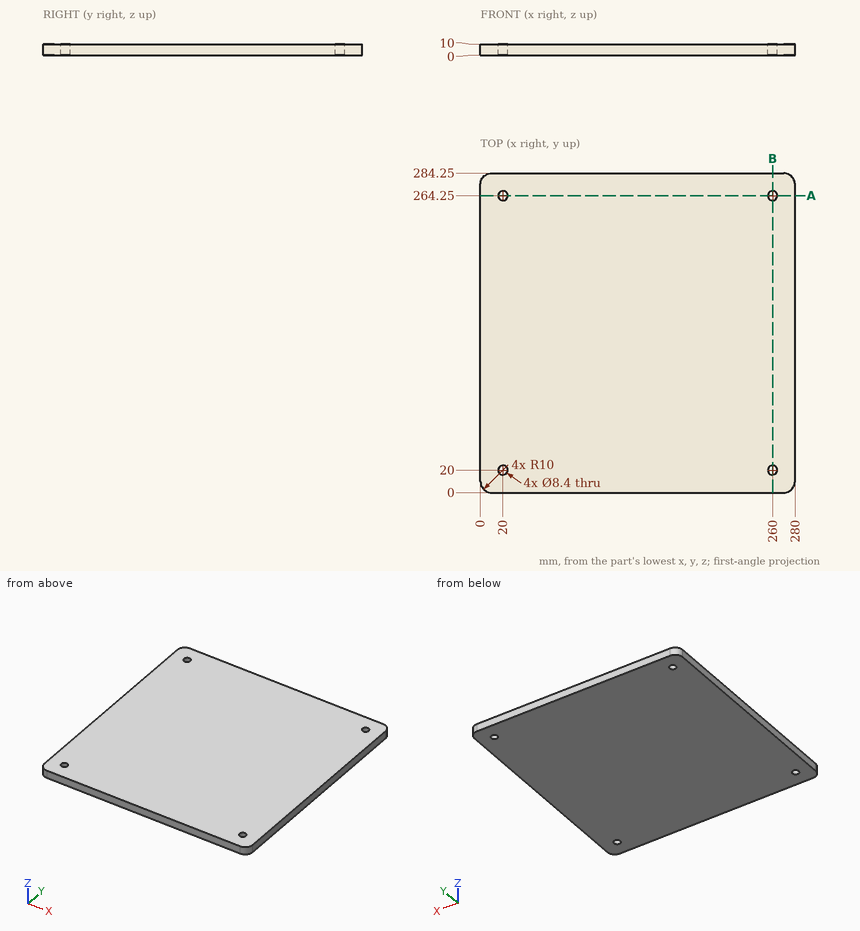
The drawing under review shows one solid part. Ordinate dimensions are in mm from its lowest x, y, z. Round coordinates to 2 decimals unless told otherwise and drop trailing zeros. Order: outer loops, then holes, each group sorted by start corner. A loop starts at its lowest first (then second) coordinate and runs counter-clockwise, first axis right, second up. Notation, with made-up numbers: M 44,-23.5 L 103,-23.5 A26 cw 103,14.5 Z; hole C -10.75,7 d11. An arc over 180 degrees is marked long. Answer as CSV lines item,"result". Start each with the question number.
1) Add section A-A (y = 264.25). Give the boundary of the cut face in (x, z).
2) For pin 1 Ø6.5 at (x, y) = (20, 20) entering from +Z, flat-tipped, find the tip position at first contact; note if it passes through.
3) Add section B-B (x = 260). Give the boundary of the cut face in (y, z).
4) Wall thickness on line 1 along X through (y, z) = (264.25, 6); line 2 along Y through (x, z) = (260, 4.5): over which ranges is each line inside the solid? List them lowest first. Write a range as [from, to].
Resolved:
1,outline,"M 0,0 L 15.8,0 L 15.8,10 L 0,10 Z; M 24.2,0 L 255.8,0 L 255.8,10 L 24.2,10 Z; M 264.2,0 L 280,0 L 280,10 L 264.2,10 Z"
2,pin 1,"through"
3,outline,"M 0,0 L 15.8,0 L 15.8,10 L 0,10 Z; M 24.2,0 L 260.05,0 L 260.05,10 L 24.2,10 Z; M 268.45,0 L 284.25,0 L 284.25,10 L 268.45,10 Z"
4,line 1,"[0, 15.8], [24.2, 255.8], [264.2, 280]"
4,line 2,"[0, 15.8], [24.2, 260.05], [268.45, 284.25]"
